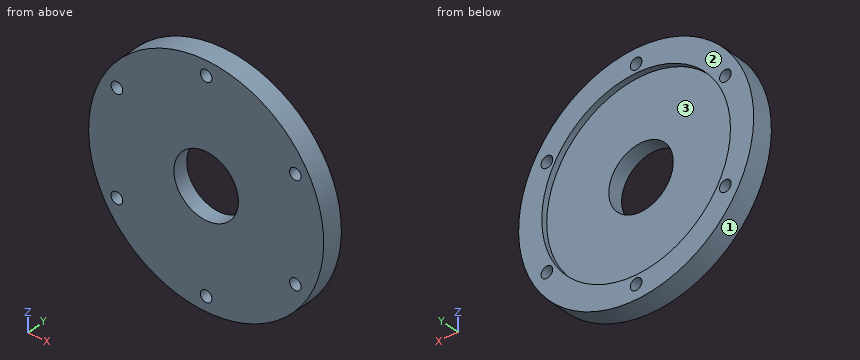
from build123d import *

# Parameters (mm, degrees)
SKETCH1_R           = 81
SKETCH1_R_2         = 22.225
SKETCH1_R_3         = 4
BOSS_EXTRUDE1_DEPTH = 14.5
SKETCH2_R           = 65
CUT_EXTRUDE1_DEPTH  = 4


with BuildPart() as part:
    # Sketch1 → Boss-Extrude1 (new body)
    with BuildSketch(Plane(origin=(0, 0, 0), x_dir=(1, 0, 0), z_dir=(0, 1, 0))):
        with Locations(Location((0, 0, 0), (0, 0, 270))):
            Circle(SKETCH1_R)
        with Locations(Location((0, 0, 0), (0, 0, 270))):
            Circle(SKETCH1_R_2, mode=Mode.SUBTRACT)
        with Locations(Location((0, 71, 0), (0, 0, 270))):
            Circle(SKETCH1_R_3, mode=Mode.SUBTRACT)
        with Locations(Location((61.487803669, 35.5, 0), (0, 0, 270))):
            Circle(SKETCH1_R_3, mode=Mode.SUBTRACT)
        with Locations(Location((61.487803669, -35.5, 0), (0, 0, 270))):
            Circle(SKETCH1_R_3, mode=Mode.SUBTRACT)
        with Locations(Location((0, -71, 0), (0, 0, 270))):
            Circle(SKETCH1_R_3, mode=Mode.SUBTRACT)
        with Locations(Location((-61.487803669, -35.5, 0), (0, 0, 270))):
            Circle(SKETCH1_R_3, mode=Mode.SUBTRACT)
        with Locations(Location((-61.487803669, 35.5, 0), (0, 0, 270))):
            Circle(SKETCH1_R_3, mode=Mode.SUBTRACT)
    extrude(amount=-BOSS_EXTRUDE1_DEPTH)

    # Sketch2 → Cut-Extrude1 (cut)
    with BuildSketch(Plane(origin=(0, 0, 0), x_dir=(1, 0, 0), z_dir=(0, 1, 0))):
        with Locations(Location((0, 0, 0), (0, 0, 270))):
            Circle(SKETCH2_R)
    extrude(amount=-CUT_EXTRUDE1_DEPTH, mode=Mode.SUBTRACT)


solid = part.part
The model under review builds one solid part; all positions refer to its coordinate system, in mm. Face numbers are marked on the shaded views. Give positions to 0.01 mm unless a question says otherwise; leave off trailing zeros. Order: outer loops, then holes, each group sorted by start corner. A loop starts at its lowest first (then second) coordinate and runs counter-clockwise, first axis right, second up. Notation, with made-up numbers: M 74,-21.75 L 118,-21.75 A24 ccw 118,-1.75 Z; hole C 41,4.25 d7. An arc over 180 degrees is marked long. Use one line per item in the form item = value. Start each with the question number.
Item 1: To check wall thickness, follow line 1 along X through (y, z) = (-1.55, 0); line 2 along X through (y, z) = (-5, -35.5); line 3 along Z through (x, y) = (2, -7.75). State the ranges of each line that lie inside material, in increasing order. Write a range as from..to.
Item 2: We need section D-D on z = 35.5. Give the boundary of the cut face in (x, y).
Item 3: Insertion check: pin 1 Ø3 at (x, y) = (30, -7.5) entering from +Z; pin 2 Ø12 at (x, z) = (-29.5, -28.5) entering from +Y; pin 3 Ø6 at (y, z) = (-8, 49) entering from -X. Each pin has a flat end and moves straight along its axis. Give the tip position at first contact, or say it passes through.
Item 4: The part is to be moulded in two halves that separate along Z. For the marked faces 1, 2 and 3, say which applies: pulls with the +Z half, pulls with the -Z half, needs draft (parallel to the pull), parting line crosses it, or undercut.
Item 5: We need section A-A on z = 0. Give the boundary of the cut face in (x, y) (3 decimals).
Item 6: We need section C-C on x = 37. Give the boundary of the cut face in (y, z).
Item 7: We need section B-B on y = -8. Give the boundary of the cut face in (x, z) (3 decimals), plus the area to 3 significant figures.
Completed:
q1.line_1 = -81..-65, 65..81
q1.line_2 = -72.81..-65.49, -57.49..57.49, 65.49..72.81
q1.line_3 = -80.98..-74.46, -67.54..-22.13, 22.13..67.54, 74.46..80.98
q2.outline = M -72.81,-14.5 L -65.49,-14.5 L -65.49,0 L -72.81,0 Z; M -57.49,-14.5 L 57.49,-14.5 L 57.49,0 L 54.45,0 L 54.45,-4 L -54.45,-4 L -54.45,0 L -57.49,0 Z; M 65.49,-14.5 L 72.81,-14.5 L 72.81,0 L 65.49,0 Z
q3.pin_1 = 75.82
q3.pin_2 = -4
q3.pin_3 = -66.67
q4.face_1 = parting line crosses it
q4.face_2 = needs draft
q4.face_3 = undercut
q5.outline = M -81,-14.5 L -22.225,-14.5 L -22.225,-4 L -65,-4 L -65,0 L -81,0 Z; M 22.225,-14.5 L 81,-14.5 L 81,0 L 65,0 L 65,-4 L 22.225,-4 Z
q6.outline = M -14.5,-72.06 L 0,-72.06 L 0,-53.44 L -4,-53.44 L -4,53.44 L 0,53.44 L 0,72.06 L -14.5,72.06 Z
q7.outline = C 0,0 d162; hole C -61.488,-35.5 d8; hole C -61.488,35.5 d8; hole C 0,0 d44.45; hole C 0,-71 d8; hole C 0,71 d8; hole C 61.488,-35.5 d8; hole C 61.488,35.5 d8
q7.area = 18,800 mm²
